Input: part model. Units: mm. Frame: model coordinates. Face numbers are marked on the shaded views. A direction names the side the tool comes from. Give positions to 0.01 mm unless a question says otherwise; leave off trailing zeros. Write each loop counter-clockwise with the first axis right and the second up, starting at its lowest first coordinate (ties: lowest second). Pieces come first, ordered by that corner, then holes. Notation, with made-up numbers: (84.5, -5.5) - (110.5, -5.5) arc R5 cw to (110.5, -1.5) - close; hole circle Ø9 at (-25, 32). An arc over 180 degrees is marked (long way). Use a Markdown table: item, result. Add a question column.
1. Mould query, pull axis Z, two halves, no side actions, for the marked faces 3, 4 and 5. Classes: released by +Z, released by -Z, zero draft, split by the parting line, or undercut.
2. Section query C-C, the plane x = 7.5. Return loops of the section in (y, z), plus the area to 3 significant figures.
3. Pin query (flat end, axial travel): pin 1 (1 mm diameter, centred on x = 1, y = -3, fed in from +Z); pin 2 (2 mm diameter, centred on y = -1.5, z = -7.5, fed in from -X); pin 3 (4.5 mm diameter, centred on x = 4, z = -2, fed in from -Y); pin 4 (6 mm diameter, centred on x = 3, z = -2, fed in from -Y). Return the tip coordinate at first contact, or that it passes through.
4. Section query A-A, the plane x = 5. Return loops of the section in (y, z), plus the area to 3 significant figures.
5. Section query B-B, the plane y = 3.75. Return loops of the section in (x, z).
6. Set-up query: the marked faces 1 and 2. Return all of +Z, -Z, +X, -X, +Y, -Y with unobstructed straight access to the full face (end or side cutting, diameter ignored); none if empty.
7. Section query D-D, the plane y = -4. Return loops of the section in (x, z), plus the area to 3 significant figures.
8. Material intervals for probe 1 along Z at (x, y) = (7, 2.5); probe 2 along Y at (x, z) = (5.5, -6.5); probe 3 along Y at (x, z) = (5, -10.4), sorted ascending.
```python
from build123d import *

# Parameters (mm, degrees)
BOSS_EXTRUDE1_DEPTH = 10
SKETCH2_R           = 1.7
CUT_EXTRUDE1_DEPTH  = 10


with BuildPart() as part:
    # Sketch1 → Boss-Extrude1 (new body)
    with BuildSketch(Plane(origin=(0, 0, 0), x_dir=(0, 0, -1), z_dir=(1, 0, 0))):
        with BuildLine():
            Line((-2.1875, 6.5), (-3.1875, 5.5))
            Line((-3.1875, 5.5), (-3.1875, 5.296875))
            Line((-3.1875, 5.296875), (-3.1875, 0))
            Line((-3.1875, 0), (-1.6875, 0))
            Line((-1.6875, 0), (-1.6875, 4))
            ThreePointArc((-1.6875, 4), (-1.394606781, 4.707106781), (-0.6875, 5))
            Line((-0.6875, 5), (8.3125, 5))
            ThreePointArc((8.3125, 5), (9.019606781, 4.707106781), (9.3125, 4))
            Line((9.3125, 4), (9.3125, -9))
            Line((9.3125, -9), (10.8125, -9))
            Line((10.8125, -9), (10.8125, 5.5))
            Line((10.8125, 5.5), (9.8125, 6.5))
            Line((9.8125, 6.5), (4.875, 6.5))
            Line((4.875, 6.5), (-2.1875, 6.5))
        make_face()
    extrude(amount=BOSS_EXTRUDE1_DEPTH)

    # Sketch2 → Cut-Extrude1 (cut)
    with BuildSketch(Plane(origin=(0, 0, -10.8125), x_dir=(-1, 0, 0), z_dir=(0, 0, -1))):
        with Locations((-5, -4)):
            Circle(SKETCH2_R)
    extrude(amount=-CUT_EXTRUDE1_DEPTH, mode=Mode.SUBTRACT)


solid = part.part
```
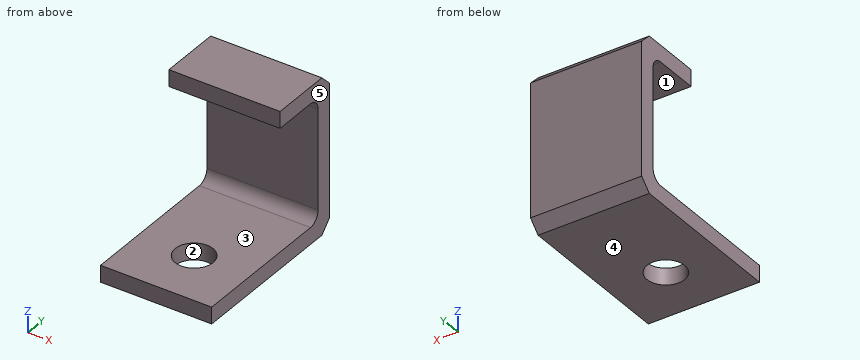
Result sheet:
| question | item | result |
|---|---|---|
| 1 | face 3 | undercut |
| 1 | face 4 | released by -Z |
| 1 | face 5 | zero draft |
| 2 | outline | (-9, -10.81) - (5.5, -10.81) - (6.5, -9.81) - (6.5, 2.19) - (5.5, 3.19) - (0, 3.19) - (0, 1.69) - (4, 1.69) arc R1 cw to (5, 0.69) - (5, -8.31) arc R1 cw to (4, -9.31) - (-9, -9.31) - close |
| 2 | area | 48.9 mm² |
| 3 | pin 1 | stops at z = -9.31 |
| 3 | pin 2 | passes through |
| 3 | pin 3 | stops at y = 5 |
| 3 | pin 4 | stops at y = 4.95 |
| 4 | outline | (-9, -10.81) - (-5.7, -10.81) - (-5.7, -9.31) - (-9, -9.31) - close; (-2.3, -10.81) - (5.5, -10.81) - (6.5, -9.81) - (6.5, 2.19) - (5.5, 3.19) - (0, 3.19) - (0, 1.69) - (4, 1.69) arc R1 cw to (5, 0.69) - (5, -8.31) arc R1 cw to (4, -9.31) - (-2.3, -9.31) - close |
| 4 | area | 43.8 mm² |
| 5 | outline | (0, -10.81) - (10, -10.81) - (10, -9.31) - (0, -9.31) - close; (0, 1.69) - (10, 1.69) - (10, 3.19) - (0, 3.19) - close |
| 6 | face 1 | +X, -X, -Y |
| 6 | face 2 | +Z, -Z |
| 7 | outline | (0, -10.81) - (3.3, -10.81) - (3.3, -9.31) - (0, -9.31) - close; (6.7, -10.81) - (10, -10.81) - (10, -9.31) - (6.7, -9.31) - close |
| 7 | area | 9.90 mm² |
| 8 | probe 1 | z = -10.81 to -9.31, 1.69 to 3.19 |
| 8 | probe 2 | y = 5 to 6.5 |
| 8 | probe 3 | y = -9 to -5.7, -2.3 to 5.91 |
